Could you check a few things on this model? Use its own coordinates, in mm. Face numbers are marked on the shaded views. A direction names the side the tool comes from. Coordinates: 2 decimals unless noted, no trailing zeros. Order: outer loops, then holes, each group sorted by start corner. A loop starts at its lowest first (then second) coordinate and runs counter-clockwise, first axis right, second up. Notation, with made-up numbers: (64.5, 45.5) - (90.5, 45.5) arc R12 ccw to (90.5, 51.5) - close; hole circle Ø8 at (4, 80). An arc over 180 degrees is marked (long way). One line per item, written item: value.
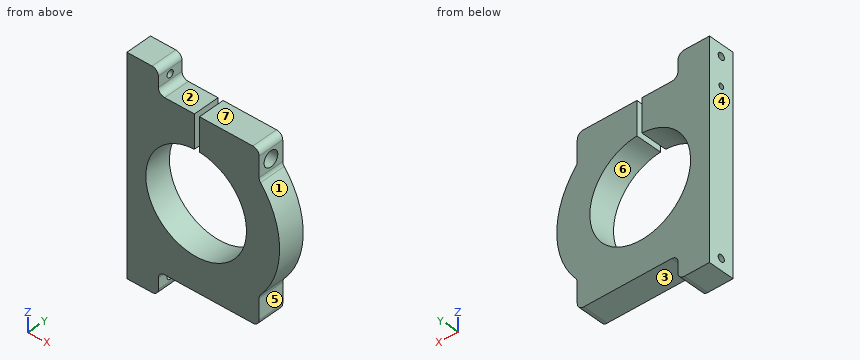
from build123d import *

# Parameters (mm, degrees)
BOSS_EXTRUDE2_DEPTH                     = 21
FILLET2_R                               = 5
M5_CLEARANCE_HOLE1_D                    = 5.5
CBORE_FOR_M5_HEX_HEAD_BOLT1_D           = 5.5
CBORE_FOR_M5_HEX_HEAD_BOLT1_DEPTH       = 47.375
CBORE_FOR_M5_HEX_HEAD_BOLT1_CBORE_D     = 12.238
CBORE_FOR_M5_HEX_HEAD_BOLT1_CBORE_DEPTH = 23.5
TAP_DRILL_FOR_M5_TAP1_D                 = 4.2
TAP_DRILL_FOR_M5_TAP1_DEPTH             = 53.625


with BuildPart() as part:
    # Sketch1 → Boss-Extrude2 (new body)
    with BuildSketch(Plane(origin=(0, 0, -219.72), x_dir=(1, 0, 0), z_dir=(0, -1, 0))):
        with BuildLine():
            Line((17.325408024, -30.717863594), (-30.049591976, -30.717863594))
            Line((-30.049591976, -30.717863594), (-30.049591976, -57.304089343))
            ThreePointArc((-30.049591976, -57.304089343), (-33.300374886, -137.212968242), (-34.049591976, -57.241503392))
            Line((-34.049591976, -57.241503392), (-34.049591976, -30.717863594))
            Line((-34.049591976, -30.717863594), (-62.674591976, -30.717863594))
            Line((-62.674591976, -30.717863594), (-62.674591976, -12.217863594))
            Line((-62.674591976, -12.217863594), (-87.674591976, -12.217863594))
            Line((-87.674591976, -12.217863594), (-87.674591976, -182.217863594))
            Line((-87.674591976, -182.217863594), (-62.674591976, -182.217863594))
            Line((-62.674591976, -182.217863594), (-62.674591976, -163.717863594))
            Line((-62.674591976, -163.717863594), (17.325408024, -163.717863594))
            Line((17.325408024, -163.717863594), (17.325408024, -140.681210221))
            ThreePointArc((17.325408024, -140.681210221), (33.575408024, -97.217863594), (17.325408024, -53.754516967))
            Line((17.325408024, -53.754516967), (17.325408024, -30.717863594))
        make_face()
    extrude(amount=BOSS_EXTRUDE2_DEPTH)

    # Fillet2
    fillet2_edges = [part.edges().sort_by_distance(p)[0] for p in [
        (-62.674591976, -10.5, -250.437863594),
        (-62.674591976, -10.5, -231.937863594),
        (-62.674591976, -10.5, -401.937863594),
        (-62.674591976, -10.5, -383.437863594),
        (17.325408024, -10.5, -383.437863594),
        (17.325408024, -10.5, -360.401210221),
        (17.325408024, -10.5, -273.474516967),
        (17.325408024, -10.5, -250.437863594),
    ]]
    fillet(fillet2_edges, radius=FILLET2_R)

    # M5 Clearance Hole1 (through all)
    with Locations(Plane(origin=(17.325408024, 0, 0), x_dir=(0, 0, -1), z_dir=(1, 0, 0))):
        with Locations((392.687863594, -10.5), (241.187863594, -10.5)):
            Hole(M5_CLEARANCE_HOLE1_D / 2)

    # CBORE for M5 Hex Head Bolt1
    with Locations(Plane(origin=(17.325408024, 0, 0), x_dir=(0, 0, -1), z_dir=(1, 0, 0))):
        with Locations((263.540774929, -10.5)):
            CounterBoreHole(CBORE_FOR_M5_HEX_HEAD_BOLT1_D / 2, CBORE_FOR_M5_HEX_HEAD_BOLT1_CBORE_D / 2, CBORE_FOR_M5_HEX_HEAD_BOLT1_CBORE_DEPTH, depth=CBORE_FOR_M5_HEX_HEAD_BOLT1_DEPTH)

    # Tap Drill for M5 Tap1
    with Locations(Plane(origin=(-34.049591976, 0, 0), x_dir=(0, 0, -1), z_dir=(1, 0, 0))):
        with Locations((263.540774929, -10.5)):
            Hole(TAP_DRILL_FOR_M5_TAP1_D / 2, depth=TAP_DRILL_FOR_M5_TAP1_DEPTH)


solid = part.part
Item 1: I want a section at C-C on z = -279.5. Please give me the cut outline in (x, y).
Conclusion:
outline: (-87.67, -21) - (-46.76, -21) - (-46.76, 0) - (-87.67, 0) - close; (-18.59, -21) - (21.98, -21) - (21.98, 0) - (-18.59, 0) - close
Item 2: I'm going to push flat-ended pins straight in: pin 1 Ø7 at (y, z) = (-6.5, -393) entering from +X; pin 2 Ø1 at (x, y) = (-8.5, -14.5) entering from -Z; pin 3 Ø2 at (y, z) = (-2.5, -279.5) entering from +X. Where does each tip first touch, or does it pass through?
Conclusion:
pin 1: x = -62.67
pin 2: z = -383.44
pin 3: x = 22.65
Item 3: I want a section at B-B on x = 10. Please give me the cut outline in (y, z), then the cut area to 3 significant figures.
Conclusion:
outline: (-21, -383.44) - (0, -383.44) - (0, -250.44) - (-21, -250.44) - close; hole circle Ø12.24 at (-10.5, -263.54)
area: 2,680 mm²
Item 4: Thinking about a two-plate mould opening in X: for the marked faces 4, 5, 6 and 7, which applies, pulls with the +X half, pulls with the -X half, needs draft (parallel to the pull), parting line crosses it, or undercut?
Conclusion:
face 4: pulls with the -X half
face 5: pulls with the +X half
face 6: undercut
face 7: needs draft
Item 5: For the marked faces 1, 2 and 3, which set-ups out of +Z, -Z, +X, -X, +Y, -Y let a thin tool reach every point of the face, with its end or its side?
Conclusion:
face 1: +X, +Y, -Y
face 2: +Z, +X, +Y, -Y
face 3: -Z, +X, +Y, -Y
Item 6: I want a section at D-D on y = -10.5. Give the number of separate pieces and of enclosed holes in the cut face, then the cut area to 3 significant figures.
Conclusion:
separate pieces: 5
enclosed holes: 0
area: 9,800 mm²
Item 7: If I drill on probe 1 along X at (y, z) = (-7.5, -267.5); probe 2 along Z at (x, y) = (-12.5, -12.25); probe 3 along Z at (x, y) = (-25, -7.5), over which ranges is the centre line in solid material (lowest first)?
Conclusion:
probe 1: -87.67 to -34.05, -30.05 to -6.17
probe 2: -383.44 to -351.48, -282.4 to -265.66, -261.42 to -250.44
probe 3: -383.44 to -356.19, -277.68 to -250.44
Item 8: I want a section at A-A on z = -354. Please give me the cut outline in (x, y).
Conclusion:
outline: (-87.67, -21) - (-47.72, -21) - (-47.72, 0) - (-87.67, 0) - close; (-17.63, -21) - (22.24, -21) - (22.24, 0) - (-17.63, 0) - close
